For this review, use the dimensioned drawing (mm, ordinates from the lowest corner) and the shaded views. A direction names the side the tool comes from. Coordinates: 2 decimals unless noted, no trailing zeros. Loops run counter-clockwise (first coordinate to the right, second up) from the corner with the lowest first, then second, coordinate; pieces in that order, holes last. Notation, with made-up numbers: M -1.75,-19.75 L 38.25,-19.75 A23 cw 38.25,1.25 Z; hole C 28,18.5 d11. An arc over 180 degrees is marked long. One line per item, written item: value.
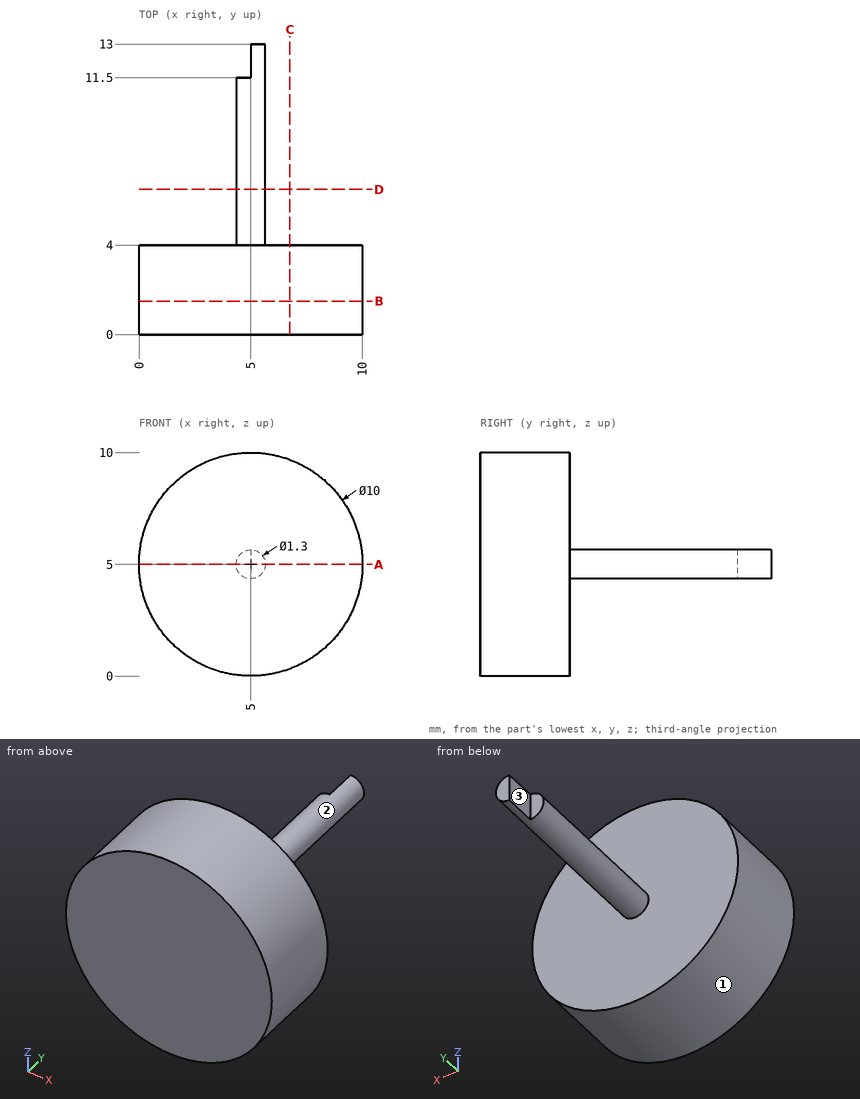
(1) We need section C-C on x = 6.75. State the section outline as (y, z) points, then the cut area to 3 significant figures.
Reply:
outline: M 0,0.32 L 4,0.32 L 4,9.68 L 0,9.68 Z
area: 37.5 mm2
(2) We need section A-A on z = 5. State the section outline as (x, y) points.
Reply:
outline: M 0,0 L 10,0 L 10,4 L 5.65,4 L 5.65,13 L 5,13 L 5,11.5 L 4.35,11.5 L 4.35,4 L 0,4 Z
(3) We need section B-B on y = 1.5. State the section outline as (x, z) points, then the cut area to 3 significant figures.
Reply:
outline: C 5,5 d10
area: 78.5 mm2
(4) We need section D-D on y = 6.5. State the section outline as (x, z) points, then the cut area to 3 significant figures.
Reply:
outline: C 5,5 d1.3
area: 1.33 mm2
(5) To check wall thickness, follow line 1 along Y through (x, z) = (2.25, 4.25); line 2 along Z through (x, y) = (5, 7.25); line 3 along X through (y, z) = (2, 3). State the ranges of each line that lie inside material, in increasing order. Write a range as [from, to].
Reply:
line 1: y = [0, 4]
line 2: z = [4.35, 5.65]
line 3: x = [0.42, 9.58]
(6) Insertion check: pin 1 (0.5 mm diameter, centred on x = 4.5, z = 5, fed in from +Y); pin 2 (1.5 mm diameter, centred on y = 2.5, z = 8, fed in from +X); pin 3 (1.5 mm diameter, centred on x = 2, y = 3.5, fed in from -Z). Each pin has a flat end and moves straight along its axis. Give the tip position at first contact, or say it passes through.
Reply:
pin 1: stops at y = 11.5
pin 2: stops at x = 9.47
pin 3: stops at z = 0.53
(7) Tool access review of the marked faces 1, 2 and 3: name each direction out of +Z, -Z, +X, -X, +Y, -Y from which nothing blocks a thin tool from reaching the whole face with its end or side.
Reply:
face 1: +Y, -Y
face 2: +Y
face 3: +Z, -Z, -X, +Y
